Read the model definition and answer for the solid it produces. Units are mm, in the model's axes. A direction names the side the tool comes from. Coordinates: 2 decimals unless noted, no trailing zeros. Order: outer loops, then holes, each group sorted by start corner. A loop starts at its lowest first (then second) coordinate and runs counter-clockwise, first axis right, second up. Notation, with made-up numbers: M 71,75 L 122,75 A11 cw 122,90 Z; hole C 71.5,43.25 d9. An arc over 180 degrees is marked long. Write each question's results on one line, items separated by ' | '.
Autodesk Inventor part; units mm, degrees
ref_plane "YZ Plane" through (0, 0, 0) normal (1, 0, 0) x (0, 1, 0)
ref_plane "XZ Plane" through (0, 0, 0) normal (0, 1, 0) x (-1, 0, 0)
ref_plane "XY Plane" through (0, 0, 0) normal (0, 0, 1) x (1, 0, 0)
sketch "Skizze1" plane through (0, 0, 0) normal (0, 1, 0) x (-1, 0, 0)
  line L0 (0, 0) -> (30, 0)
  line L1 (30, 0) -> (30, 40)
  line L2 (30, 40) -> (0, 40)
  line L3 (0, 40) -> (0, 0)
  circle A0 centre (15, 33) radius 2.55
  circle A1 centre (15, 7) radius 2.55
  dimension "d0" = 30
  dimension "d1" = 40
  dimension "d2" = 5.1
  dimension "d3" = 5.1
  dimension "d4" = 7
  dimension "d5" = 7
  dimension "d6" = 15
  dimension "d7" = 15
extrude "Baseplate" add sketch "Skizze1" along normal blind 5
sketch "Skizze2" plane through (0, 0, 40) normal (1, 0, 0) x (0, 0, -1)
  arc A0 (27.2284, 5) -> (12.7716, 5) centre (20, 7) ccw
  line L0 (40, 0) -> (40, 5)
  line L1 (0, 5) -> (40, 5)
  line L2 (12.7716, 5) -> (27.2284, 5)
  line L3 (40, 5) -> (0, 5)
  dimension "d10" = 15
  dimension "d12" = 20
  dimension "d13" = 2
extrude "Rounding" add sketch "Skizze2" against normal up to surface (30 mm away)
sketch "Skizze3" plane through (0, 0, 40) normal (1, 0, 0) x (0, 0, -1)
  line L0 (40, 0) -> (40, 5)
  line L1 (27.2284, 5) -> (40, 5)
  circle A0 centre (20, 7) radius 4.05
  dimension "d17" = 20
  dimension "d18" = 2
  dimension "d19" = 8.1
hole "Sensor" at (0, 7, 20) direction (-1, 0, 0) diameter 12.2 end through all
fillet "Rundung1" radius 4 2 edges at (-15, 5, 27.2284) (-15, 5, 12.7716)
fillet "Rundung2" radius 2 2 edges at (-15, 5, 0) (-15, 5, 40)
chamfer "Fase1" distance 1 angle 45 18 edges at (0, 1.5, 40) (0, 4.4142, 39.4142) (0, 5, 34.6624) (0, 5.9355, 28.754) (0, 5.9355, 11.246) (0, 14.5, 20) (0, 5, 5.3376) (0, 4.4142, 0.5858) (0, 1.5, 0) (-30, 5.9355, 28.754) (-30, 5.9355, 11.246) (-30, 14.5, 20) (-30, 5, 34.6624) (-30, 4.4142, 39.4142) (-30, 1.5, 40) (-30, 5, 5.3376) (-30, 4.4142, 0.5858) (-30, 1.5, 0)
equation "\"d3\" = d2"
equation "\"d5\" = d4"
properties part number "Prox_Z_3030"
(1) Given pin 1 (1.5 mm diameter, centred on x = -23, z = 10.5, fed in from +Y); pin 2 (1 mm diameter, centred on y = 3, z = 22, fed in from -X); pin 3 (7.5 mm diameter, centred on x = -17.5, z = 33.5, fed in from +Y); pin 4 (7.5 mm diameter, centred on x = -9.5, z = 6, fed in from +Y), each flat-ended and moving along its own axis, determine where each tip first touches the part or whether it passes through.
Conclusion:
pin 1: y = 5.94 | pin 2: through | pin 3: y = 5.32 | pin 4: y = 5.15
(2) For faces 5 (the flat face through (-15, 5, 4)), 6 (the flat face through (-29.5, 4.5, 34.6)), 7 (the flat face through (-0.5, 1.5, 39.5)), 8 (the flat face through (-29.5, 4.5, 5.3)), 9 (the flat face through (-0.5, 4.5, 34.6)), determine the directions among +Z, -Z, +X, -X, +Y, -Y from which every point of the face is accessible in a straight line to the end or side of a thin tool.
Conclusion:
face 5: -Z, +X, -X, +Y | face 6: +Z, -X, +Y | face 7: +Z, +X, +Y, -Y | face 8: -Z, -X, +Y | face 9: +Z, +X, +Y
(3) Straight lines are drawn through the part: line 1 (Z direction, x = -15, y = 2.25); line 2 (X direction, y = 3.85, z = 33); line 3 (Z direction, x = -15, y = 3.25). For each, find the intervals that lie inside material, in ascending order.
Conclusion:
line 1: 0 to 4.45, 9.55 to 16.17, 23.83 to 30.45, 35.55 to 40 | line 2: -30 to -17.55, -12.45 to 0 | line 3: 0.02 to 4.45, 9.55 to 15.19, 24.81 to 30.45, 35.55 to 39.98
(4) The part is cut by section D-D, the plane z = 20. Write down the section's boundary in (x, y).
Conclusion:
outline: M -30,0 L 0,0 L 0,0.9 L -30,0.9 Z; M -30,13.1 L 0,13.1 L 0,13.5 L -1,14.5 L -29,14.5 L -30,13.5 Z
(5) The part is cut by section B-B, the plane z = 33. Write down the section's boundary in (x, y).
Conclusion:
outline: M -30,0 L -17.55,0 L -17.55,5 L -29,5 L -30,4 Z; M -12.45,0 L 0,0 L 0,4 L -1,5 L -12.45,5 Z
(6) The part is cut by section C-C, the plane x = -23.75. Write down the section's boundary in (y, z), then the cut area to 3 significant figures.
Conclusion:
outline: M 0,0 L 3,0 A2 ccw 5,2 L 5,8.68 A4 cw 8.3,12.61 A7.5 ccw 8.3,27.39 A4 cw 5,31.32 L 5,38 A2 ccw 3,40 L 0,40 Z; hole C 7,20 d12.2 | area: 206 mm²
(7) The part is cut by section A-A, the plane x = -15. Write down the section's boundary in (y, z), then the cut area to 3 significant figures.
Conclusion:
outline: M 0,0 L 3,0 A2 ccw 5,2 L 5,4.45 L 0,4.45 Z; M 0,9.55 L 5.1,9.55 A4 cw 8.3,12.61 A7.5 ccw 8.3,27.39 A4 cw 5.1,30.45 L 0,30.45 Z; M 0,35.55 L 5,35.55 L 5,38 A2 ccw 3,40 L 0,40 Z; hole C 7,20 d12.2 | area: 154 mm²
(8) The mould has two halves that part along Z. Classify faces 1 (the flat face through (-29.5, 1.5, 0.5)), 2 (the conical face through (-29.6, 4, 38.98)), 3 (the cylindrical face through (-12.452, 2.513, 6.888)), 4 (the flat face through (-15, 0, 20)): pulls with the +Z half, pulls with the -Z half, needs draft (parallel to the pull), parting line crosses it, or undercut.
Conclusion:
face 1: pulls with the -Z half | face 2: pulls with the +Z half | face 3: undercut | face 4: needs draft
